For this review, take the finished solid that the model builds, in its own axes (mm). A direction names the side the tool comes from. Round coordinates to 2 decimals unless told otherwise and drop trailing zeros. Order: outer loops, then holes, each group sorted by start corner. A loop starts at its lowest first (then second) coordinate and runs counter-clockwise, first axis right, second up. Notation, with made-up numbers: M 54.5,73 L 63.5,73 A19 cw 63.5,79 Z; hole C 34,28 d11. An arc over 180 degrees is marked long. Answer as a JSON object with one key per item and string values.
from build123d import *

# Parameters (mm, degrees)
F1_DEPTH = 984
F4_DEPTH = 5
F7_DEPTH = 5
F8_R     = 2


# Not quite as in the source:
# - a feature names something its author has since deleted; it is built from what else it names


with BuildPart() as f1:
    # F0 (on Right) → F1 (new body)
    with BuildSketch(Plane.YZ):
        Polygon((-295, 0), (0, 0), (0, 430), (-5, 430), (-5, 5), (-290, 5), (-290, 430), (-295, 430), align=None)
    extrude(amount=F1_DEPTH)

    # F3 (on offset) → F4 (join)
    with BuildSketch(Plane.YZ.offset(200)):
        Polygon((-230, 0), (-5, 0), (-5, 360), align=None)
    extrude(amount=F4_DEPTH)

    # F6 (on offset) → F7 (join)
    with BuildSketch(Plane.YZ.offset(805)):
        Polygon((-290, 360), (-290, 5), (-65, 5), align=None)
    extrude(amount=F7_DEPTH)

    # F8
    f8_edges = [f1.edges().sort_by_distance(p)[0] for p in [
        (492, 0, 0),
        (492, -295, 0),
    ]]
    fillet(f8_edges, radius=F8_R)


solid = f1.part
1) Add section A-A on y = -45. State the section outline as (x, z) points, and give its area (4 significant figures).
Geometry check:
{"outline": "M 0,0 L 984,0 L 984,5 L 205,5 L 205,296 L 200,296 L 200,5 L 0,5 Z", "area": "6,375 mm²"}
2) Machinability: for faces 4 (the flat face through (205, -68, 106)), 5 (the flat face through (200, -68, 106)), 6 (the flat face through (485, -295, 219)), 7 (the flat face through (807.465, -175.925, 180.015)), 8 (the flat face through (485, -150, 0)), which of the approach directions +Z, -Z, +X, -X, +Y, -Y give a long, thin tool a straight path to every point of the face, cutting with its end or side? Answer none if there is none.
Geometry check:
{"face 4": "+Z", "face 5": "+Z, -X", "face 6": "+Z, -Z, +X, -X, -Y", "face 7": "+Z, +X", "face 8": "-Z, +X, -X, +Y, -Y"}
3) Insertion check: P1, Ø2, axis at x = 544, y = -83.5, coming from the +Z side; P2, Ø1, axis at y = -211, z = 126, coming from the +X side. Each pin has a flat end and moves straight along its axis. Give the tip position at first contact, or say it passes through.
Geometry check:
{"P1": "stops at z = 5", "P2": "stops at x = 810"}
4) Mouldability with a two-part tool opening along Y and no side actions: class faces 1 (the flat face through (485, -5, 220)), 2 (the flat face through (485, 0, 213)), 3 (the flat face through (0, -290.2, 216)) as +Y half, -Y half, draft (parallel to the pull), parting line (faces both ways), or undercut.
Geometry check:
{"face 1": "undercut", "face 2": "+Y half", "face 3": "draft"}
5) Add section B-B on z = 171.5. State the section outline as (x, y) points, and give its area (3 significant figures).
Geometry check:
{"outline": "M 0,-295 L 984,-295 L 984,-290 L 810,-290 L 810,-170.53 L 805,-170.53 L 805,-290 L 0,-290 Z; M 0,-5 L 200,-5 L 200,-122.81 L 205,-122.81 L 205,-5 L 984,-5 L 984,0 L 0,0 Z", "area": "11,000 mm²"}
6) Add section D-D on z = 286.5. State the section outline as (x, y) points, and give its area (3 significant figures).
Geometry check:
{"outline": "M 0,-295 L 984,-295 L 984,-290 L 810,-290 L 810,-243.42 L 805,-243.42 L 805,-290 L 0,-290 Z; M 0,-5 L 200,-5 L 200,-50.94 L 205,-50.94 L 205,-5 L 984,-5 L 984,0 L 0,0 Z", "area": "10,300 mm²"}
7) For L1, parallel to Y at x = 84.5, z = 88; L2, parallel to X at y = -157, z = 90.5; L3, parallel to X at y = -105, z = 195, list the stretches that pass through material, from the lowest coordinate up.
Geometry check:
{"L1": "y = -295 to -290, -5 to 0", "L2": "x = 200 to 205, 805 to 810", "L3": "x = 200 to 205"}
8) Add section C-C on x = 296.5. State the section outline as (y, z) points, and give its area (3 significant figures).
Geometry check:
{"outline": "M -295,2 A2 ccw -293,0 L -2,0 A2 ccw 0,2 L 0,430 L -5,430 L -5,5 L -290,5 L -290,430 L -295,430 Z", "area": "5,720 mm²"}
